Input: part model. Units: mm. Frame: model coordinates. A direction names the side the tool comes from. Coordinates: 2 decimals unless noted, no trailing zeros. Write each loop counter-clockwise with the first axis right and the second up, starting at its lowest first coordinate (ties: lowest second). Pieces come first, ordered by that corner, then holes. Notation, with made-up numbers: M 32,61.25 L 59,61.25 A20 ccw 59,84.25 Z; hole C 55.5,-24 d6. An arc over 180 degrees is marked long. Answer as a JSON object with one key per item and string values. Group by question number.
from build123d import *

# Parameters (mm, degrees)
F0_R      = 13.5
F1_DEPTH  = 17.2
F2_R      = 14.5
F3_DEPTH  = 11.5
F4_R      = 1.75
F4_W      = 2.95831
F4_H      = 12
F5_DEPTH  = 0.5
F6_R      = 3
F7_DEPTH  = 1.5
F8_R      = 1.5
F9_DEPTH  = 10
F10_W     = 2.236068
F10_H     = 1.743455
F11_DEPTH = 8


with BuildPart() as f1:
    # F0 (on Top) → F1 (new body)
    with BuildSketch(Plane.XY):
        Circle(F0_R)
    extrude(amount=-F1_DEPTH)

    # F2 (on face) → F3 (join)
    with BuildSketch(Plane.XY):
        Circle(F2_R)
    extrude(amount=F3_DEPTH)

    # F4 (on face) → F5 (join, symmetric)
    with BuildSketch(Plane.XY.offset(11.5)):
        with BuildLine():
            Line((-14.5, -6), (-14.5, 6))
            Line((-14.5, 6), (-20.038462, 3.692308))
            ThreePointArc((-20.038462, 3.692308), (-22.5, 0), (-20.038462, -3.692308))
            Line((-20.038462, -3.692308), (-14.5, -6))
        make_face()
        with Locations((-18.5, 0)):
            Circle(F4_R, mode=Mode.SUBTRACT)
        with Locations((-13.020845, 0)):
            Rectangle(F4_W, F4_H)
        with BuildLine():
            ThreePointArc((20.038462, -3.692308), (22.5, 0), (20.038462, 3.692308))
            Line((20.038462, 3.692308), (14.5, 6))
            Line((14.5, 6), (14.5, -6))
            Line((14.5, -6), (20.038462, -3.692308))
        make_face()
        with Locations((18.5, 0)):
            Circle(F4_R, mode=Mode.SUBTRACT)
        with Locations((13.020845, 0)):
            Rectangle(F4_W, F4_H)
    extrude(amount=F5_DEPTH, both=True)

    # F6 (on face) → F7 (join)
    with BuildSketch(Plane.XY.offset(11.5)):
        with Locations((0, 6.5)):
            Circle(F6_R)
    extrude(amount=F7_DEPTH)

    # F8 (on face) → F9 (join)
    with BuildSketch(Plane.XY.offset(13)):
        with Locations((0, 6.5)):
            Circle(F8_R)
    extrude(amount=F9_DEPTH)

    # F10 (on face) → F11 (cut)
    with BuildSketch(Plane.XY.offset(23)):
        with Locations((0, 8.371727)):
            Rectangle(F10_W, F10_H)
    extrude(amount=-F11_DEPTH, mode=Mode.SUBTRACT)


solid = f1.part
Q1. Section D-D, the plane z = 14. Return the cut outline in (x, y), and give its area (3 significant figures).
Q2. Line query: line 1 (Z direction, x = -16, y = 2.25); line 2 (Z direction, x = -10, y = -5.5); line 3 (Y direction, x = -18.5, z = 11.45). Output: solid intervals per line, ascending. Write a range as from..to.
Q3. Section A-A, the plane y = 0. Return the cut outline in (x, z).
Q4. Access query for faces 4 (the cylindrical face through (-2.93, -13.18, -8.48)), 5 (the flat face through (1, 8, 13)), 6 (the flat face through (16, 0, 12)), 7 (the flat face through (0, 7.5, 19)), 8 (the flat face through (-16, 0, 12)). Directions: +Z, -Z, +X, -X, +Y, -Y. A direction counts if a zero-diameter tool reaches every point of the face in a straight line with its end or side. Return the directions, or none.
Q5. Draft query along X for faces 1 (the flat face through (0, 6, 23)), 2 (the cylindrical face through (-20.25, 0.08, 11.49)), 3 (the cylindrical face through (0, 5, 18)). Return one class per face: released by +X, released by -X, zero draft, split by the parting line, or undercut.
Q6. Section B-B, the plane x = 0. Return the cut outline in (y, z), and give its area (3 significant figures).
Q7. Pin query (flat end, axial travel): pin 1 Ø0.5 at (x, z) = (-12.5, 11.5) entering from -Y; pin 2 Ø1 at (x, y) = (-4.5, 10) entering from +Z; pin 3 Ø6 at (x, z) = (4, -9) entering from +Y; pin 4 Ø12 at (x, z) = (-2, 17) entering from -Y. Return the tip coordinate at first contact, or that it passes through.
Q8. Section C-C, the plane x = 18.5. Return the cut outline in (y, z).
Filled in:
{
 "1": {"outline": "C 0,6.5 d3", "area": "7.07 mm^2"},
 "2": {"line 1": "11..12", "line 2": "-17.2..11.5", "line 3": "-4.33..-1.75, 1.75..4.33"},
 "3": {"outline": "M -22.5,11 L -20.25,11 L -20.25,12 L -22.5,12 Z; M -16.75,11 L -14.5,11 L -14.5,0 L -13.5,0 L -13.5,-17.2 L 13.5,-17.2 L 13.5,0 L 14.5,0 L 14.5,11 L 16.75,11 L 16.75,12 L 11.54,12 L 11.54,11.5 L -11.54,11.5 L -11.54,12 L -16.75,12 Z; M 20.25,11 L 22.5,11 L 22.5,12 L 20.25,12 Z"},
 "4": {"face 4": "-Z", "face 5": "+Z", "face 6": "+Z, +X, +Y, -Y", "face 7": "+Z, +X, -X, +Y", "face 8": "+Z, -X, +Y, -Y"},
 "5": {"face 1": "zero draft", "face 2": "undercut", "face 3": "split by the parting line"},
 "6": {"outline": "M -14.5,0 L -13.5,0 L -13.5,-17.2 L 13.5,-17.2 L 13.5,0 L 14.5,0 L 14.5,11.5 L 9.5,11.5 L 9.5,13 L 8,13 L 8,15 L 7.5,15 L 7.5,23 L 5,23 L 5,13 L 3.5,13 L 3.5,11.5 L -14.5,11.5 Z", "area": "833 mm^2"},
 "7": {"pin 1": "y = -7.76", "pin 2": "z = 11.5", "pin 3": "y = 13.46", "pin 4": "y = -14.5"},
 "8": {"outline": "M -4.33,11 L -1.75,11 L -1.75,12 L -4.33,12 Z; M 1.75,11 L 4.33,11 L 4.33,12 L 1.75,12 Z"}
}
